from build123d import *

# Parameters (mm, degrees)
SKETCH1_W           = 38.1
SKETCH1_H           = 63.5
BOSS_EXTRUDE1_DEPTH = 63.5
SKETCH2_W           = 60.96
SKETCH2_H           = 60.96
CUT_EXTRUDE1_DEPTH  = 12.7
LPATTERN1_COUNT     = 2
LPATTERN1_PITCH     = 25.4
FILLET1_R           = 7
FILLET2_R           = 7


with BuildPart() as part:
    # Sketch1 → Boss-Extrude1 (new body)
    with BuildSketch(Plane(origin=(0, 0, 0), x_dir=(1, 0, 0), z_dir=(0, 1, 0))):
        Rectangle(SKETCH1_W, SKETCH1_H)
    extrude(amount=BOSS_EXTRUDE1_DEPTH)

    # Sketch2 → Cut-Extrude1 (cut)
    with BuildSketch(Plane(origin=(19.05, 0, 0), x_dir=(0, 0, -1), z_dir=(1, 0, 0))):
        with Locations((0, 31.75)):
            Rectangle(SKETCH2_W, SKETCH2_H)
    cut_extrude1 = extrude(amount=-CUT_EXTRUDE1_DEPTH, mode=Mode.SUBTRACT)

    # LPattern1: Cut-Extrude1 ×2
    with Locations(*[(-i * LPATTERN1_PITCH, 0, 0) for i in range(1, LPATTERN1_COUNT)]):
        add(cut_extrude1, mode=Mode.SUBTRACT)

    # Fillet1
    # the kernel refuses this fillet: 7 mm, written as the material it takes off along each edge
    with BuildSketch(Plane(origin=(19.05, 63.5, -49.25), x_dir=(0, -1, 0), z_dir=(0, 0, 1)), Plane(origin=(-19.05, 63.5, 49.25), x_dir=(0, -1, 0), z_dir=(0, 0, -1))) as fillet1_piece_1:
        with BuildLine():
            CenterArc((FILLET1_R, -FILLET1_R), FILLET1_R, 90, 90)
            Line((0, -FILLET1_R), (0, 0))
            Line((0, 0), (FILLET1_R, 0))
        make_face()
    extrude(amount=98.5, mode=Mode.SUBTRACT)

    # Fillet2
    # the kernel refuses this fillet: 7 mm, written as the material it takes off along each edge
    with BuildSketch(Plane(origin=(-19.05, 0, 49.25), x_dir=(1, 0, 0), z_dir=(0, 0, -1)), Plane(origin=(19.05, 0, -49.25), x_dir=(-1, 0, 0), z_dir=(0, 0, 1))) as fillet2_piece_1:
        with BuildLine():
            CenterArc((FILLET2_R, -FILLET2_R), FILLET2_R, 90, 90)
            Line((0, -FILLET2_R), (0, 0))
            Line((0, 0), (FILLET2_R, 0))
        make_face()
    extrude(amount=98.5, mode=Mode.SUBTRACT)


solid = part.part
Part model, mm, in its own coordinate system. A direction names the side the tool comes from. Round coordinates to 2 decimals unless told otherwise and drop trailing zeros. Write each loop counter-clockwise with the first axis right and the second up, starting at its lowest first coordinate (ties: lowest second). Pieces come first, ordered by that corner, then holes. Notation, with made-up numbers: M 27.5,71.25 L 75.5,71.25 A21 cw 75.5,85.25 Z; hole C -26,63 d9. An arc over 180 degrees is marked long. Return JSON: item names as keys, results as strings. Group by question number.
(1) Saw through at A-A on x = -9. Write the cut outline in (y, z), then the cut area to 3 significant figures.
(2) Which spindle directions (+Z, -Z, +X, -X, +Y, -Y) get a long thin tool onto all of the face, cutting with end or side? Do faces 4 (the face through (-13, 31, 30.48)), 5 (the face through (6.35, 32, 0)), 6 (the face through (-13.79, 0.22, 0.44)). Say none if no direction does.
(3) Drill centre lines: probe 1 along Y at (x, z) = (10, 5.5); probe 2 along Z at (x, y) = (16, 47.5); probe 3 along X at (y, z) = (30.5, 14.5). Where is each one in solid material? Low to high.
(4) Two-plate mould, pull along Y, no slides. Class faces 1 (the face through (0, 0, 0)), 2 (the face through (0, 31, 31.75)), 3 (the face through (-11, 1.27, 0)): +Y half, -Y half, draft (parallel to the pull), parting line (faces both ways), or undercut.
(5) Pin check, flat tips, straight feed: pin 1 Ø1 at (y, z) = (32, -6) entering from +X; pin 2 Ø1 at (y, z) = (23.5, -22.5) entering from -X. Stop position of each tip, or through.
(6) Saw through at C-C on y = 9.5. Write the cut outline in (x, z).
(7) Saw through at B-B on z = 19. Write the cut outline in (x, y), then the cut area to 3 significant figures.
Returned:
{
 "1": {"outline": "M 0,-31.75 L 63.5,-31.75 L 63.5,31.75 L 0,31.75 Z; hole M 1.27,-30.48 L 62.23,-30.48 L 62.23,30.48 L 1.27,30.48 Z", "area": "316 mm²"},
 "2": {"face 4": "-X", "face 5": "+X", "face 6": "+Z, -Z, -X, -Y"},
 "3": {"probe 1": "0 to 1.27, 62.23 to 63.5", "probe 2": "-31.75 to -30.48, 30.48 to 31.75", "probe 3": "-6.35 to 6.35"},
 "4": {"face 1": "-Y half", "face 2": "draft", "face 3": "undercut"},
 "5": {"pin 1": "x = 6.35", "pin 2": "x = -6.35"},
 "6": {"outline": "M -19.05,-31.75 L 19.05,-31.75 L 19.05,-30.48 L 6.35,-30.48 L 6.35,30.48 L 19.05,30.48 L 19.05,31.75 L -19.05,31.75 L -19.05,30.48 L -6.35,30.48 L -6.35,-30.48 L -19.05,-30.48 Z"},
 "7": {"outline": "M -16.07,1.27 A7 ccw -12.05,0 L 12.05,0 A7 ccw 16.07,1.27 L 6.35,1.27 L 6.35,62.23 L 16.07,62.23 A7 ccw 12.05,63.5 L -12.05,63.5 A7 ccw -16.07,62.23 L -6.35,62.23 L -6.35,1.27 Z", "area": "849 mm²"}
}
